```python
from build123d import *

# Parameters (mm, degrees)
F0_R     = 1.85
F3_DEPTH = 2
F4_R     = 1.85
F4_R_2   = 1.6
F5_DEPTH = 1
F6_R     = 1.15
F7_DEPTH = 2


with BuildPart() as f2:
    # F1 (on Front) → F2 (revolve)
    with BuildSketch(Plane.XZ):
        with BuildLine():
            Line((0, 0), (0, 1.5))
            Line((0, 1.5), (-1.85, 1.5))
            ThreePointArc((-1.85, 1.5), (-2.2059803133, 0.75), (-1.85, 0))
            Line((-1.85, 0), (0, 0))
        make_face()
    revolve(axis=Axis((0, 0, 0.75), (0, 0, -1)))

    # F0 (on Top) → F3 (join)
    with BuildSketch(Plane.XY):
        Circle(F0_R)
    extrude(amount=-F3_DEPTH)

    # F4 (on face) → F5 (join)
    with BuildSketch(Plane(origin=(0, 0, -2), x_dir=(1, 0, 0), z_dir=(0, 0, -1))):
        with BuildLine():
            ThreePointArc((-2.2001077956, -2.526267145), (1.3878290393, -3.0490048471), (3.35, 0))
            ThreePointArc((3.35, 0), (1.3878290393, 3.0490048471), (-2.2001077956, 2.526267145))
            ThreePointArc((-2.2001077956, 2.526267145), (-3.35, 0), (-2.2001077956, -2.526267145))
        make_face()
        Circle(F4_R, mode=Mode.SUBTRACT)
        with BuildLine():
            ThreePointArc((-8, 0), (-8.3008157574, 1.3093526739), (-9.142936283, 2.3561227369))
            ThreePointArc((-9.142936283, 2.3561227369), (-14, 0), (-9.142936283, -2.3561227369))
            ThreePointArc((-9.142936283, -2.3561227369), (-8.3008157574, -1.3093526739), (-8, 0))
        make_face()
        with Locations((-11, 0)):
            Circle(F4_R_2, mode=Mode.SUBTRACT)
        with BuildLine():
            ThreePointArc((-2.2001077956, -2.526267145), (-3.35, 0), (-2.2001077956, 2.526267145))
            ThreePointArc((-2.2001077956, 2.526267145), (-5.640853454, 1.1897478328), (-9.142936283, 2.3561227369))
            ThreePointArc((-9.142936283, 2.3561227369), (-8.3008157574, 1.3093526739), (-8, 0))
            ThreePointArc((-8, 0), (-8.3008157574, -1.3093526739), (-9.142936283, -2.3561227369))
            ThreePointArc((-9.142936283, -2.3561227369), (-5.640853454, -1.1897478328), (-2.2001077956, -2.526267145))
        make_face()
        Circle(F4_R)
    extrude(amount=F5_DEPTH)

    # F6 (on face) → F7 (cut)
    with BuildSketch(Plane.XY.offset(1.5)):
        Circle(F6_R)
    extrude(amount=-F7_DEPTH, mode=Mode.SUBTRACT)


solid = f2.part
```
Model file for the job. Use its own axes, mm. A direction names the side the tool comes from. Round coordinates to 2 decimals unless told otherwise and drop trailing zeros. Write each loop counter-clockwise with the first axis right and the second up, starting at its lowest first coordinate (ties: lowest second). Pieces come first, ordered by that corner, then holes. Notation, with made-up numbers: M -10,65 L 26,65 A12 ccw 26,88 Z; hole C -20.5,-21.5 d2. An arc over 180 degrees is marked long. Put each result on its own line as item: value.
Item 1: Cut at D-D (z = -1.05). List the corners of the cut face in (x, y), and give its area (3 significant figures).
Responses:
outline: C 0,0 d3.7
area: 10.8 mm²
Item 2: Mould opens along X. For faces 1 (the cylindrical face through (-0.401, -1.806, -0.986)), 2 (the flat face through (-5, 0, -2)), 3 (the cylindrical face through (-5.59, -1.19, -2.49)) say: +X half, -X half, draft (parallel to the pull), parting line (faces both ways), or undercut.
Responses:
face 1: parting line
face 2: draft
face 3: undercut
Item 3: Flat gauge pins, fed straight in: P1, Ø1, axis at x = -3.5, y = -1, coming from the +Z side; P2, Ø1, axis at x = -5.5, z = 0, coming from the +Y side; P3, Ø2, axis at y = -0.5, z = 0, coming from the -X side. Where does each tip first touch, or does it go through?
Responses:
P1: z = -2
P2: through
P3: x = -2.21
Item 4: Cut at A-A (x = -11). List the corners of the cut face in (y, z), and give its area (3 significant figures).
Responses:
outline: M -3,-3 L -1.6,-3 L -1.6,-2 L -3,-2 Z; M 1.6,-3 L 3,-3 L 3,-2 L 1.6,-2 Z
area: 2.80 mm²
Item 5: Tool access for faces 4 (the flat face through (0, 0, -0.5)), 5 (the flat face through (-4, 0, -3)): list every direction of +Z, -Z, +X, -X, +Y, -Y with a clear straight run to the whole face (end or side of a thin tool).
Responses:
face 4: +Z
face 5: -Z, +X, -X, +Y, -Y
Item 6: Probe L1, parallel to Y at x = -11, z = -2.3; L2, parallel to Z at x = -3, y = -1; L3, parallel to Y at x = 0, z = 0.65. List the from-to ranges inside material, lowest first. Write a range as from..to.
Responses:
L1: -3..-1.6, 1.6..3
L2: -3..-2
L3: -2.2..-1.15, 1.15..2.2
Item 7: Cut at B-B (x = 0). List the corners of the cut face in (y, z), and give its area (3 significant figures).
Responses:
outline: M -3.35,-3 L 3.35,-3 L 3.35,-2 L 1.85,-2 L 1.85,0 A0.97 ccw 1.85,1.5 L 1.15,1.5 L 1.15,-0.5 L -1.15,-0.5 L -1.15,1.5 L -1.85,1.5 A0.97 ccw -1.85,0 L -1.85,-2 L -3.35,-2 Z
area: 15.8 mm²
Item 8: Cut at C-C (z = -2.5). List the corners of the cut face in (x, y), and give its area (3 significant figures).
Responses:
outline: M -9.14,-2.36 A5.44 cw -2.2,-2.53 A3.35 ccw long -2.2,2.53 A5.44 cw -9.14,2.36 A3 ccw long Z; hole C -11,0 d3.2
area: 69.7 mm²
